Input: part model. Units: mm. Frame: model coordinates. A direction names the side the tool comes from. Round coordinates to 2 decimals unless told otherwise and drop trailing zeros. Write each loop counter-clockwise with the first axis right and the second up, starting at its lowest first coordinate (ties: lowest second). Pieces come first, ordered by that corner, then holes. Notation, with made-up numbers: (-7, -11) -> (2, -11) arc R28 ccw to (2, 24) -> close; hole circle Ø8 at (-18, 64.5). An arc over 180 degrees is marked (long way). Write item = value, one per line.
```python
from build123d import *

# Parameters (mm, degrees)
SKETCH1_R           = 11
SKETCH1_R_2         = 1
BOSS_EXTRUDE1_DEPTH = 6
SKETCH2_R           = 4
CUT_EXTRUDE1_DEPTH  = 5.5
SKETCH3_R           = 6
BOSS_EXTRUDE2_DEPTH = 5
SKETCH6_R           = 1
CUT_EXTRUDE2_DEPTH  = 6
SKETCH6_3_R         = 1.5
SKETCH6_3_R_2       = 1
CUT_EXTRUDE3_DEPTH  = 2


with BuildPart() as part:
    # Sketch1 → Boss-Extrude1 (new body)
    with BuildSketch(Plane(origin=(0, 0, 0), x_dir=(1, 0, 0), z_dir=(0, 1, 0))):
        with Locations(Location((0, 0, 0), (0, 0, 270))):
            Circle(SKETCH1_R)
        with Locations(Location((0, 8, 0), (0, 0, 270))):
            Circle(SKETCH1_R_2, mode=Mode.SUBTRACT)
        with Locations(Location((5.656854249, 5.656854249, 0), (0, 0, 270))):
            Circle(SKETCH1_R_2, mode=Mode.SUBTRACT)
        with Locations(Location((8, 0, 0), (0, 0, 270))):
            Circle(SKETCH1_R_2, mode=Mode.SUBTRACT)
        with Locations(Location((5.656854249, -5.656854249, 0), (0, 0, 270))):
            Circle(SKETCH1_R_2, mode=Mode.SUBTRACT)
        with Locations(Location((0, -8, 0), (0, 0, 270))):
            Circle(SKETCH1_R_2, mode=Mode.SUBTRACT)
        with Locations(Location((-5.656854249, -5.656854249, 0), (0, 0, 270))):
            Circle(SKETCH1_R_2, mode=Mode.SUBTRACT)
        with Locations(Location((-8, 0, 0), (0, 0, 270))):
            Circle(SKETCH1_R_2, mode=Mode.SUBTRACT)
        with Locations(Location((-5.656854249, 5.656854249, 0), (0, 0, 270))):
            Circle(SKETCH1_R_2, mode=Mode.SUBTRACT)
    extrude(amount=BOSS_EXTRUDE1_DEPTH)

    # Sketch2 → Cut-Extrude1 (cut)
    with BuildSketch(Plane.XZ):
        with Locations(Location((0, 0, 0), (0, 0, 270))):
            Circle(SKETCH2_R)
    extrude(amount=-CUT_EXTRUDE1_DEPTH, mode=Mode.SUBTRACT)

    # Sketch3 → Boss-Extrude2 (add)
    with BuildSketch(Plane(origin=(0, 6, 0), x_dir=(1, 0, 0), z_dir=(0, 1, 0))):
        with Locations(Location((0, 0, 0), (0, 0, 270))):
            Circle(SKETCH3_R)
        with BuildLine():
            ThreePointArc((1.5, 0), (-0.866025404, -1.224744871), (-0.5, 1.414213562))
            Line((-0.5, 1.414213562), (-0.5, 2.514213562))
            Line((-0.5, 2.514213562), (0.5, 2.514213562))
            Line((0.5, 2.514213562), (0.5, 1.414213562))
            ThreePointArc((0.5, 1.414213562), (1.224744871, 0.866025404), (1.5, 0))
        make_face(mode=Mode.SUBTRACT)
    extrude(amount=BOSS_EXTRUDE2_DEPTH)

    # Sketch6 → Cut-Extrude2 (cut)
    with BuildSketch(Plane.XY.offset(6)):
        with Locations((0, 8.5)):
            Circle(SKETCH6_R)
    extrude(amount=-CUT_EXTRUDE2_DEPTH, mode=Mode.SUBTRACT)

    # Sketch6_3 → Cut-Extrude3 (cut)
    with BuildSketch(Plane.XY.offset(6)):
        with Locations((0, 8.5)):
            Circle(SKETCH6_3_R)
        with Locations((0, 8.5)):
            Circle(SKETCH6_3_R_2, mode=Mode.SUBTRACT)
    extrude(amount=-CUT_EXTRUDE3_DEPTH, mode=Mode.SUBTRACT)


solid = part.part
```
1) Cut plane B-B (z = -8). Return the cut outline in (x, y), and give its area (3 significant figures).
Solutions:
outline = (-7.55, 0) -> (-1, 0) -> (-1, 6) -> (-7.55, 6) -> close; (1, 0) -> (7.55, 0) -> (7.55, 6) -> (1, 6) -> close
area = 78.6 mm^2
2) First-contact query: P1, Ø2.5, axis at x = 0, y = 8.5, coming from the +Z side; P2, Ø1, axis at x = -1.5, z = -2, coming from the -Y side; P3, Ø1.2, axis at y = 8, z = -2, coming from the +X side; P4, Ø1.6, axis at x = -5.66, z = 5.66, coming from the -Y side. Flat tips, straight axial feed; report the tip coordinate or a pass-through.
Solutions:
P1 = 4
P2 = 5.5
P3 = 5.83
P4 = through
3) Cut plane C-C (x = -8). Return the cut outline in (y, z), and give its area (3 significant figures).
Solutions:
outline = (0, -7.55) -> (6, -7.55) -> (6, -1) -> (0, -1) -> close; (0, 1) -> (6, 1) -> (6, 7.55) -> (0, 7.55) -> close
area = 78.6 mm^2
4) Draft query along Z for faces 1 (the face through (1.802, 8.465, 5.723)), 2 (the face through (0, 8, -2.514)), 3 (the face through (-5, 0, 0)). Return one class per face: +Z half, -Z half, draft (parallel to the pull), parting line (faces both ways), or undercut.
Solutions:
face_1 = parting line
face_2 = undercut
face_3 = draft
5) Line query: L1, parallel to X at y = 3.05, z = 0; L2, parallel to Z at x = 5.75, y = 1.25. Output: solid intervals per line, ascending. Write a range as from..to.
Solutions:
L1 = -11..-9, -7..-4, 4..7, 9..11
L2 = -9.38..-6.65, -4.66..4.66, 6.65..9.38
6) Cut plane D-D (y = 8). Return the cut outline in (x, z).
Solutions:
outline = (-1.41, 4) -> (-1.41, 5.83) arc R6 ccw (long way) to (1.41, 5.83) -> (1.41, 4) -> (0.87, 4) -> (0.87, 1.22) arc R1.5 cw to (0.5, -1.41) -> (0.5, -2.51) -> (-0.5, -2.51) -> (-0.5, -1.41) arc R1.5 cw to (-0.87, 1.22) -> (-0.87, 4) -> close
7) Cut plane A-A (x = 0). Count the separate pieces of the cut face and the enclosed holes in it, and give its area (3 significant figures).
Solutions:
separate_pieces = 4
enclosed_holes = 0
area = 92.9 mm^2
8) Access query for faces 4 (the face through (-0.5, 8, -2)), 5 (the face through (-3.905, 2.712, 0.867)), 6 (the face through (0.46, 7.61, 2.58)), 7 (the face through (-7, 3, 0)), 8 (the face through (-1.2, 11, 1.2)). Directions: +Z, -Z, +X, -X, +Y, -Y. A direction counts if a zero-diameter tool reaches every point of the face in a straight line with its end or side. Return the directions, or none.
Solutions:
face_4 = +Y
face_5 = -Y
face_6 = +Z
face_7 = +Y, -Y
face_8 = +Z, -Z, +X, -X, +Y
